The figure shows three views and two pictorial views of one solid part (mm, origin at its lowest corner). Answer the questions. Coordinates: 2 decimals unless noted, no trailing zeros. Write each loop counter-clockwise with the first axis right and the second up, starting at its lowest first coordinate (ties: lowest second). Pieces come first, ordered by that corner, then holes.
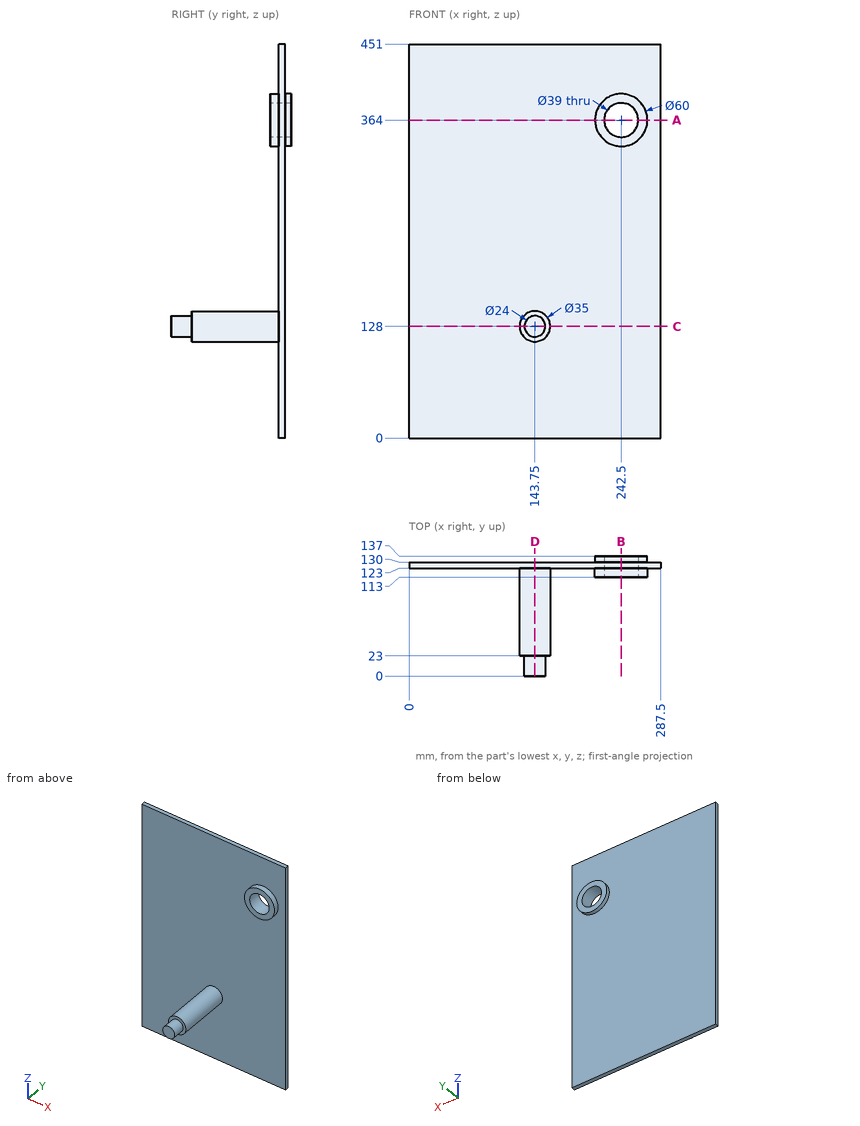
Q1. The part is cut by section A-A, the plane z = 364. Write down the section's boundary in (x, y), then the cut area to 3 significant figures.
Answers below:
outline: (0, 123) - (212.5, 123) - (212.5, 113) - (223, 113) - (223, 137) - (212.5, 137) - (212.5, 130) - (0, 130) - close; (262, 113) - (272.5, 113) - (272.5, 123) - (287.5, 123) - (287.5, 130) - (272.5, 130) - (272.5, 137) - (262, 137) - close
area: 2,100 mm2
Q2. The part is cut by section D-D, the plane x = 143.75. Write down the section's boundary in (y, z), then the cut area to 3 significant figures.
Answers below:
outline: (0, 116) - (23, 116) - (23, 110.5) - (123, 110.5) - (123, 0) - (130, 0) - (130, 451) - (123, 451) - (123, 145.5) - (23, 145.5) - (23, 140) - (0, 140) - close
area: 7,210 mm2
Q3. The part is cut by section C-C, the plane z = 128. Write down the section's boundary in (x, y).
Answers below:
outline: (0, 123) - (126.25, 123) - (126.25, 23) - (131.75, 23) - (131.75, 0) - (155.75, 0) - (155.75, 23) - (161.25, 23) - (161.25, 123) - (287.5, 123) - (287.5, 130) - (0, 130) - close
Q4. The part is cut by section B-B, the plane x = 242.5. Write down the section's boundary in (y, z).
Answers below:
outline: (113, 334) - (123, 334) - (123, 0) - (130, 0) - (130, 334) - (137, 334) - (137, 344.5) - (113, 344.5) - close; (113, 383.5) - (137, 383.5) - (137, 394) - (130, 394) - (130, 451) - (123, 451) - (123, 394) - (113, 394) - close
Q5. Find the intervals of material crossed by probe 1 along Z at (x, y) = (242, 126); probe 2 along Z at (x, y) = (242.5, 122.5); probe 3 along Y at (x, z) = (41, 27.5), in increasing order.
Answers below:
probe 1: z = 0 to 344.51, 383.49 to 451
probe 2: z = 334 to 344.5, 383.5 to 394
probe 3: y = 123 to 130
Q6. Given pin 1 (5 mm diameter, centred on x = 62, z = 57.5, fed in from -Y); pin 2 (3 mm diameter, centred on x = 41.5, z = 329, fed in from +Y); pin 3 (10 mm diameter, centred on x = 162.5, y = 43.5, fed in from +Z), each flat-ended and moving along its own axis, determine where each tip first touches the part or whether it passes through.
Answers below:
pin 1: stops at y = 123
pin 2: stops at y = 130
pin 3: stops at z = 138.83
